CAD build for the part. Positions are in the model's coordinates, mm. A direction names the side the tool comes from. Give positions to 0.01 mm unless a question says otherwise; leave off trailing zeros. Order: outer loops, then holes, each group sorted by start corner. A loop starts at its lowest first (then second) coordinate and runs counter-clockwise, first axis right, second up.
```python
from build123d import *

# Parameters (mm, degrees)
F1_DEPTH = 6.35
F2_R     = 2.54
F3_DEPTH = 6.35
F4_W     = 8.89
F4_H     = 10.16
F5_DEPTH = 2.54
F6_R     = 2.54
F7_DEPTH = 25.4


with BuildPart() as f1:
    # F0 (on Top) → F1 (new body)
    with BuildSketch(Plane.XY):
        Polygon((0, 63.5), (0, 0), (89.802561, -89.802561), (121.552561, -58.052561), (63.5, 0), (63.5, 16.51), (16.51, 16.51), (16.51, 63.5), align=None)
    extrude(amount=F1_DEPTH)

    # F2 (on face) → F3 (cut)
    with BuildSketch(Plane.XY.offset(6.35)):
        with Locations((12.7, 50.8)):
            Circle(F2_R)
        with Locations((49.53, 12.7)):
            Circle(F2_R)
        with Locations((12.7, 12.7)):
            Circle(F2_R)
    extrude(amount=-F3_DEPTH, mode=Mode.SUBTRACT)

    # F4 (on face) → F5 (join)
    with BuildSketch(Plane.XY.offset(6.35)):
        with Locations((12.065, 50.8)):
            Rectangle(F4_W, F4_H)
    extrude(amount=F5_DEPTH)

    # F6 (on face) → F7 (cut)
    with BuildSketch(Plane.XY.offset(8.89)):
        with Locations((12.7, 50.8)):
            Circle(F6_R)
    extrude(amount=-F7_DEPTH, mode=Mode.SUBTRACT)


solid = f1.part
```
Item 1: Tool access for faces 5 (the face through (12.37, 15.22, 3.22)), 6 (the face through (40, 16.51, 3)): list every direction of +Z, -Z, +X, -X, +Y, -Y with a clear straight run to the whole face (end or side of a thin tool).
Item 2: Slice it at A-A (y = 12.7). Give the cut face in (x, z), and give its area (3 significant figures).
Item 3: Slice it at D-D (y = 50.8). Give the cut face in (x, z).
Item 4: Slice it at C-C (x = 49.53). Give the cut face in (y, z).
Item 5: Slice it at B-B (z = 3.25). Give the cut face in (x, y), and give its area (3 significant figures).
Item 6: Wall check: L1, parallel to Y at x = 12.7, z = 1.5; L2, parallel to X at y = 28.5, z = 3.75; L3, parallel to Z at x = 52.5, y = -45. Give the ranges that are in metal, low to high.
Item 7: Two-plate mould, pull along Y, no slides. Class faces 1 (the face through (12.15, 48.32, 4.51)), 2 (the face through (51.953, 13.463, 3.219)), 3 (the face through (105.455, -74.15, 3.131)), 4 (the face through (16.51, 40, 3)): released by +Y, released by -Y, zero draft, split by the parting line, or undercut.
Item 8: Drop flat-ended pins along their axis: pin 1 Ø4 at (x, z) = (49.5, 4) entering from +Y; pin 2 Ø1 at (x, z) = (27.5, 6.5) entering from -Y; pin 3 Ø3 at (y, z) = (6.5, 4.5) entering from +X. Give the stop position or say it passes through.
A:
1. face 5: +Z, -Z
1. face 6: +Z, -Z, +X, +Y
2. outline: (0, 0) - (10.16, 0) - (10.16, 6.35) - (0, 6.35) - close; (15.24, 0) - (46.99, 0) - (46.99, 6.35) - (15.24, 6.35) - close; (52.07, 0) - (63.5, 0) - (63.5, 6.35) - (52.07, 6.35) - close
2. area: 339 mm2
3. outline: (0, 0) - (10.16, 0) - (10.16, 8.89) - (7.62, 8.89) - (7.62, 6.35) - (0, 6.35) - close; (15.24, 0) - (16.51, 0) - (16.51, 8.89) - (15.24, 8.89) - close
4. outline: (-49.53, 0) - (10.16, 0) - (10.16, 6.35) - (-49.53, 6.35) - close; (15.24, 0) - (16.51, 0) - (16.51, 6.35) - (15.24, 6.35) - close
5. outline: (0, 0) - (89.8, -89.8) - (121.55, -58.05) - (63.5, 0) - (63.5, 16.51) - (16.51, 16.51) - (16.51, 63.5) - (0, 63.5) - close; hole circle Ø5.08 at (12.7, 12.7); hole circle Ø5.08 at (12.7, 50.8); hole circle Ø5.08 at (49.53, 12.7)
5. area: 6,460 mm2
6. L1: y = -12.7 to 10.16, 15.24 to 48.26, 53.34 to 63.5
6. L2: x = 0 to 16.51
6. L3: z = 0 to 6.35
7. face 1: undercut
7. face 2: undercut
7. face 3: released by -Y
7. face 4: zero draft
8. pin 1: stops at y = 16.51
8. pin 2: stops at y = -27.98
8. pin 3: stops at x = 63.5
